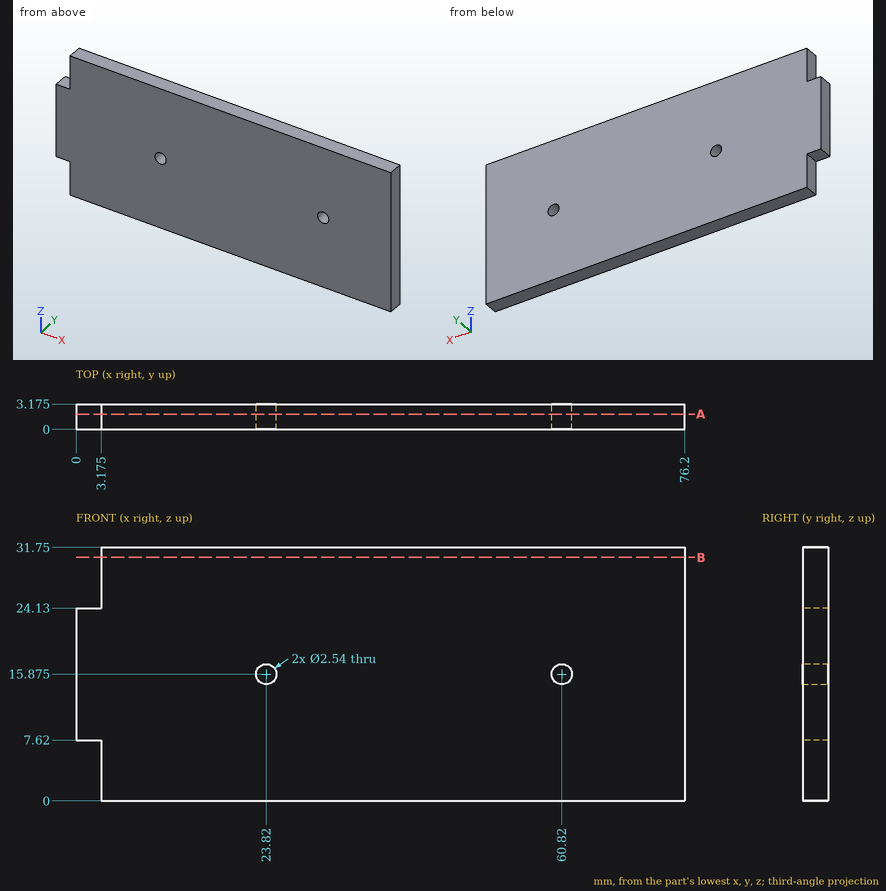
Job drawing, mm, ordinate dimensions from the low corner. One solid piece. Coordinates: 2 decimals unless noted, no trailing zeros. Write each loop counter-clockwise with the first axis right and the second up, starting at its lowest first coordinate (ties: lowest second). Pieces come first, ordered by that corner, then holes. Notation, with made-up numbers: (-28, 74) - (13, 74) arc R8 ccw to (13, 85) - close; hole circle Ø7 at (40, 5). An arc over 180 degrees is marked (long way). Use a Markdown table: item, result. Add a question column.
Item 1: Band-saw the part on A-A, the plane y = 1.9. Give the number of separate pieces and of enclosed holes in the cut face, and give its area (3 significant figures).
Item 2: Band-saw the part on B-B, the plane z = 30.5. Give the cut face in (x, y) (1 decimal), and give its area (3 significant figures).
Item 3: Drill centre lines: L1, parallel to X at y = 2.65, z = 16; L2, parallel to X at y = 0.7, z = 4 (1 decimal); L3, parallel to Z at x = 24.5, y = 1. Where is each one in solid material? Low to high. Write a range as from..to.
Item 4: Flat gauge pins, fed straight in: pin 1 (8 mm diameter, centred on x = 66.5, z = 19, fed in from -Y); pin 2 (1.6 mm diameter, centred on y = 2, z = 2.5, fed in from -X) (3 decimals). Where does each tip first touch, or does it go through?
Numbers:
| question | item | result |
|---|---|---|
| 1 | separate pieces | 1 |
| 1 | enclosed holes | 2 |
| 1 | area | 2,360 mm2 |
| 2 | outline | (3.2, 0) - (76.2, 0) - (76.2, 3.2) - (3.2, 3.2) - close |
| 2 | area | 232 mm2 |
| 3 | L1 | 0..22.56, 25.08..59.56, 62.08..76.2 |
| 3 | L2 | 3.2..76.2 |
| 3 | L3 | 0..14.8, 16.95..31.75 |
| 4 | pin 1 | y = 0 |
| 4 | pin 2 | x = 3.175 |
